The drawing under review shows one solid part. Ordinate dimensions are in mm from its lowest x, y, z. A direction names the side the tool comes from. Round coordinates to 2 decimals unless told otherwise and drop trailing zeros. Order: outer loops, then holes, each group sorted by start corner. A loop starts at its lowest first (then second) coordinate and runs counter-clockwise, first axis right, second up.
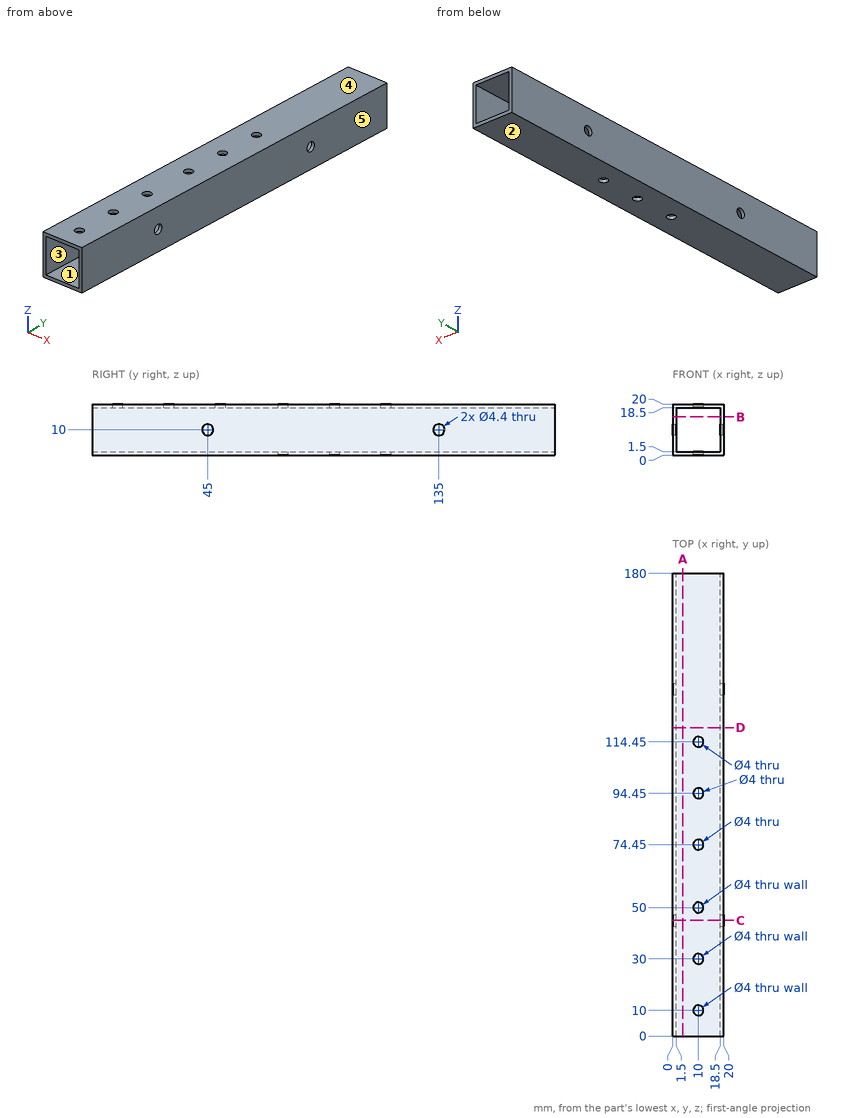
Q1. Wall thickness on line 1 (Y direction, x = 0.4, z = 10); line 2 (Z direction, x = 18.25, y = 20): over which ranges is each line inside the solid? List them lowest first.
Q2. Take a section at A-A, the plane x = 4. State the section outline as (y, z) points, plus the area to 3 significant figures.
Q3. Tool access review of the marked faces 1 and 2: name each direction out of +Z, -Z, +X, -X, +Y, -Y from which nothing blocks a thin tool from reaching the whole face with its end or side.
Q4. Take a section at B-B, the plane z = 15. State the section outline as (x, y) points, plus the area to 3 significant figures.
Q5. Take a section at C-C, the plane y = 45. State the section outline as (x, z) points, plus the area to 3 significant figures.
Q6. Mouldability with a two-part tool opening along Z and no side actions: class the marked faces 3, 4 and 5 as +Z half, -Z half, draft (parallel to the pull), parting line (faces both ways), or undercut.
Q7. Take a section at D-D, the plane y = 120. State the section outline as (x, z) points.
Working result:
1. line 1: y = 0 to 42.8, 47.2 to 132.8, 137.2 to 180
1. line 2: z = 0 to 1.5, 18.5 to 20
2. outline: (0, 0) - (180, 0) - (180, 1.5) - (0, 1.5) - close; (0, 18.5) - (180, 18.5) - (180, 20) - (0, 20) - close
2. area: 540 mm2
3. face 1: +Y, -Y
3. face 2: -Z, +X, -X, +Y, -Y
4. outline: (0, 0) - (1.5, 0) - (1.5, 180) - (0, 180) - close; (18.5, 0) - (20, 0) - (20, 180) - (18.5, 180) - close
4. area: 540 mm2
5. outline: (0, 0) - (20, 0) - (20, 7.8) - (18.5, 7.8) - (18.5, 1.5) - (1.5, 1.5) - (1.5, 7.8) - (0, 7.8) - close; (0, 12.2) - (1.5, 12.2) - (1.5, 18.5) - (18.5, 18.5) - (18.5, 12.2) - (20, 12.2) - (20, 20) - (0, 20) - close
5. area: 97.8 mm2
6. face 3: undercut
6. face 4: +Z half
6. face 5: draft
7. outline: (0, 0) - (20, 0) - (20, 20) - (0, 20) - close; hole (1.5, 1.5) - (18.5, 1.5) - (18.5, 18.5) - (1.5, 18.5) - close
